Print and shaded views of the part. All mm, measured from the part's lowest x, y and z. A direction names the side the tool comes from. Round coordinates to 2 decimals unless told otherwise and drop trailing zeros. Loops run counter-clockwise (first coordinate to the right, second up) from the corner with the lowest first, then second, coordinate; pieces in that order, holes last. Notation, with made-up numbers: (7.5, 34) -> (58.5, 34) arc R30 cw to (58.5, 62) -> close; hole circle Ø2 at (-21, -40). An arc over 180 degrees is marked (long way). Answer as CSV lines item,"result".
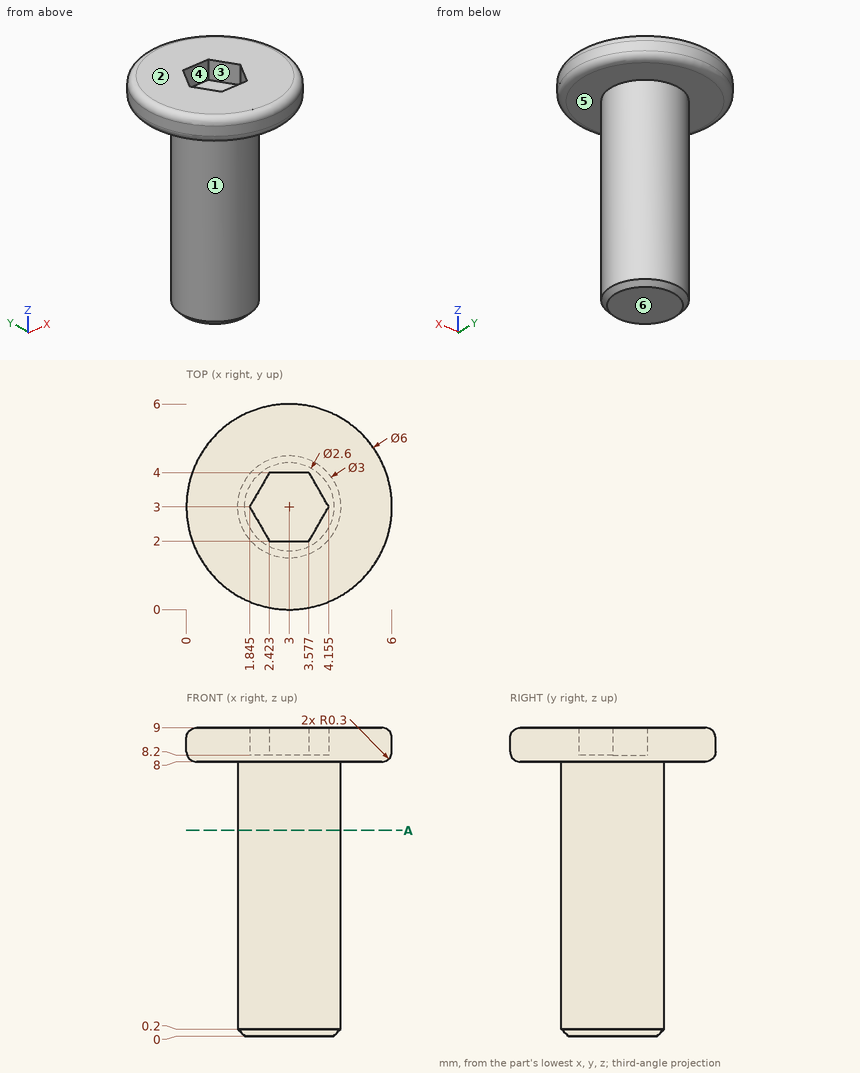
Q1. Slice it at A-A, the plane z = 6. Give the cut face in (x, y).
Results:
outline,"circle Ø3 at (3, 3)"
Q2. Tool access for the marked faces 4, 5 and 6: list every direction of +Z, -Z, +X, -X, +Y, -Y with a clear straight run to the whole face (end or side of a thin tool).
Results:
face 4,"+Z"
face 5,"-Z"
face 6,"-Z, +X, -X, +Y, -Y"
Q3. Drop flat-ended pins along their axis: pin 1 Ø2 at (x, z) = (5, 3.5) entering from +Y; pin 2 Ø0.6 at (x, z) = (3.5, 8.5) entering from +Y; pin 3 Ø1 at (x, z) = (5.5, 7) entering from +Y. Give the stop position or say it passes through.
Results:
pin 1,"y = 4.12"
pin 2,"y = 5.99"
pin 3,"through"
Q4. Two-plate mould, pull along X, no slides. Class the marked faces 1, 2 and 3: pulls with the +X half, pulls with the -X half, needs draft (parallel to the pull), parting line crosses it, or undercut.
Results:
face 1,"parting line crosses it"
face 2,"needs draft"
face 3,"undercut"
Q5. Probe L1, parallel to Z at x = 3.75, y = 1.5; L2, parallel to Y at x = 3.25, z = 8.5; L3, parallel to Y at x = 2, z = 8.25 (1 decimal). List the from-to ranges inside material, lowest first. Write a range as [from, to].
Results:
L1,"[8, 9]"
L2,"[0.01, 2], [4, 5.99]"
L3,"[0.2, 2.7], [3.3, 5.8]"
